Here's how the part is built. I have some questions about the finished solid (model axes, mm). A direction names the side the tool comes from. Coordinates: 2 decimals unless noted, no trailing zeros. Write each loop counter-clockwise with the first axis right and the second up, starting at its lowest first coordinate (ties: lowest second). Pieces come first, ordered by that corner, then holes.
Item 1: Please list where these lines run through material, in increasing order: line 1 (Y direction, x = 20, z = 2.3); line 2 (X direction, y = -10.5, z = 3.65); line 3 (Z direction, x = -14.5, y = -19.5).
Item 2: I'm going to push flat-ended pins straight in: P1, Ø2, axis at x = 4, z = 3, coming from the +Y side; P2, Ø1, axis at y = 5.5, z = 4, coming from the -X side; P3, Ø2, axis at x = 2.5, z = 2.5, coming from the +Y side; P4, Ø10, axis at x = -18.5, y = 14.5, coming from the -Z side. Where does each tip first touch, or does it pass through?
Item 3: I want a section at B-B (y = 4.5). Please give me the cut outline in (x, z).
Item 4: For faces 5 (the face through (2, 2, 4.5)), 6 (the face through (0, -11.067, 2)), 7 (the face through (4, 22, 3)), which set-ups out of +Z, -Z, +X, -X, +Y, -Y let a thin tool reach every point of the face, with its end or its side?
Item 5: If we mould it in two halves opening along X, with no side actions, what happens to faces 1 (the face through (0, -7.667, 2)), 2 (the face through (-0.336, -20.563, 2.282)), 3 (the face through (20.956, 6.599, 3.74)), 4 (the face through (-0.4, -11.5, 0))? For each: pulls with the +X half, pulls with the -X half, needs draft (parallel to the pull), parting line crosses it, or undercut.
Item 6: I want a section at D-D (y = 14.05). Please give me the cut outline in (x, z), and give its area (3 significant figures).
Item 7: I want a section at A-A (z = 3.7). Count the separate pieces of the cut face and the enclosed holes in it, and give its area (3 significant figures).
from build123d import *

# Parameters (mm, degrees)
SKETCH1_R           = 26.67
SKETCH1_R_2         = 21.971
SKETCH1_R_3         = 18.5
BOSS_EXTRUDE1_DEPTH = 3
SKETCH1_3_R         = 21.971
SKETCH1_3_R_2       = 18.5
BOSS_EXTRUDE2_DEPTH = 4.5
SKETCH2_R           = 1.55
CUT_EXTRUDE2_DEPTH  = 38.984573184


with BuildPart() as part:
    # Sketch1 → Boss-Extrude1 (new body)
    # profile 1 of 3: a face of its own
    with BuildSketch(Plane.XY):
        Circle(SKETCH1_R)
        Circle(SKETCH1_R_2, mode=Mode.SUBTRACT)
    # profile 2 of 3: a face of its own
    with BuildSketch(Plane.XY):
        Circle(SKETCH1_R_2)
        Circle(SKETCH1_R_3, mode=Mode.SUBTRACT)
    # profile 3 of 3: a face of its own
    with BuildSketch(Plane.XY):
        Circle(SKETCH1_R_3)
    extrude(amount=BOSS_EXTRUDE1_DEPTH)

    # Sketch1<3> → Boss-Extrude2 (add)
    # profile 1 of 2: a face of its own
    with BuildSketch(Plane.XY):
        Circle(SKETCH1_3_R)
        Circle(SKETCH1_3_R_2, mode=Mode.SUBTRACT)
    # profile 2 of 2: a face of its own
    with BuildSketch(Plane.XY):
        Circle(SKETCH1_3_R_2)
    extrude(amount=BOSS_EXTRUDE2_DEPTH)

    # Sketch2 → Cut-Extrude2 (cut, through all)
    with BuildSketch(Plane.XY.offset(4.5)):
        with Locations((0, 19.05)):
            Circle(SKETCH2_R)
        with Locations((0, -19.05)):
            Circle(SKETCH2_R)
        with BuildLine():
            Line((-12.86468033, 12.35), (12.86468033, 12.35))
            ThreePointArc((12.86468033, 12.35), (14.56468033, 14.05), (12.86468033, 15.75))
            Line((12.86468033, 15.75), (-12.86468033, 15.75))
            ThreePointArc((-12.86468033, 15.75), (-14.56468033, 14.05), (-12.86468033, 12.35))
        make_face()
        with BuildLine():
            Line((-16.588190244, 7.666666667), (16.588190244, 7.666666667))
            ThreePointArc((16.588190244, 7.666666667), (18.288190244, 9.366666667), (16.588190244, 11.066666667))
            Line((16.588190244, 11.066666667), (-16.588190244, 11.066666667))
            ThreePointArc((-16.588190244, 11.066666667), (-18.288190244, 9.366666667), (-16.588190244, 7.666666667))
        make_face()
        with BuildLine():
            Line((-18.465342913, 2.983333333), (18.465342913, 2.983333333))
            ThreePointArc((18.465342913, 2.983333333), (20.165342913, 4.683333333), (18.465342913, 6.383333333))
            Line((18.465342913, 6.383333333), (-18.465342913, 6.383333333))
            ThreePointArc((-18.465342913, 6.383333333), (-20.165342913, 4.683333333), (-18.465342913, 2.983333333))
        make_face()
        with BuildLine():
            Line((-19.05, -1.7), (19.05, -1.7))
            ThreePointArc((19.05, -1.7), (20.75, 0), (19.05, 1.7))
            Line((19.05, 1.7), (-19.05, 1.7))
            ThreePointArc((-19.05, 1.7), (-20.75, 0), (-19.05, -1.7))
        make_face()
        with BuildLine():
            Line((-18.465342913, -6.383333333), (18.465342913, -6.383333333))
            ThreePointArc((18.465342913, -6.383333333), (20.165342913, -4.683333333), (18.465342913, -2.983333333))
            Line((18.465342913, -2.983333333), (-18.465342913, -2.983333333))
            ThreePointArc((-18.465342913, -2.983333333), (-20.165342913, -4.683333333), (-18.465342913, -6.383333333))
        make_face()
        with BuildLine():
            Line((-16.588190244, -11.066666667), (16.588190244, -11.066666667))
            ThreePointArc((16.588190244, -11.066666667), (18.288190244, -9.366666667), (16.588190244, -7.666666667))
            Line((16.588190244, -7.666666667), (-16.588190244, -7.666666667))
            ThreePointArc((-16.588190244, -7.666666667), (-18.288190244, -9.366666667), (-16.588190244, -11.066666667))
        make_face()
        with BuildLine():
            Line((-12.86468033, -15.75), (12.86468033, -15.75))
            ThreePointArc((12.86468033, -15.75), (14.56468033, -14.05), (12.86468033, -12.35))
            Line((12.86468033, -12.35), (-12.86468033, -12.35))
            ThreePointArc((-12.86468033, -12.35), (-14.56468033, -14.05), (-12.86468033, -15.75))
        make_face()
    extrude(amount=-CUT_EXTRUDE2_DEPTH, mode=Mode.SUBTRACT)


solid = part.part
Answer:
1. line 1: y = -17.64 to -5.41, -3.95 to -1.41, 1.41 to 3.95, 5.41 to 17.64
1. line 2: x = -19.3 to -17.86, 17.86 to 19.3
1. line 3: z = 0 to 3
2. P1: stops at y = 26.5
2. P2: stops at x = -21.39
2. P3: stops at y = 26.63
2. P4: stops at z = 0
3. outline: (-26.29, 0) - (-20.16, 0) - (-20.16, 4.5) - (-21.51, 4.5) - (-21.51, 3) - (-26.29, 3) - close; (20.16, 0) - (26.29, 0) - (26.29, 3) - (21.51, 3) - (21.51, 4.5) - (20.16, 4.5) - close
4. face 5: +Z, +X, -X, +Y, -Y
4. face 6: +Z, -Z
4. face 7: +Z
5. face 1: undercut
5. face 2: undercut
5. face 3: parting line crosses it
5. face 4: needs draft
6. outline: (-22.67, 0) - (-14.56, 0) - (-14.56, 4.5) - (-16.89, 4.5) - (-16.89, 3) - (-22.67, 3) - close; (14.56, 0) - (22.67, 0) - (22.67, 3) - (16.89, 3) - (16.89, 4.5) - (14.56, 4.5) - close
6. area: 55.6 mm2
7. separate pieces: 1
7. enclosed holes: 9
7. area: 657 mm2
